from build123d import *

# Parameters (mm, degrees)
SKETCH1_W           = 127
SKETCH1_H           = 57.15
SKETCH1_R           = 14.3002
SKETCH1_R_2         = 2.38125
BOSS_EXTRUDE1_DEPTH = 3.175
SKETCH2_R           = 2.38125
CUT_EXTRUDE1_DEPTH  = 3.175
FILLET1_R           = 5.08
SKETCH3_R           = 3.175
CUT_EXTRUDE2_DEPTH  = 3.175
SKETCH4_R           = 16.51
CUT_EXTRUDE3_DEPTH  = 7.62
SKETCH5_W           = 76.2
SKETCH5_H           = 12.7
BOSS_EXTRUDE2_DEPTH = 3.175
FILLET2_R           = 5.08
SKETCH6_W           = 25.4
SKETCH6_H           = 5.08
BOSS_EXTRUDE3_DEPTH = 3.175
FILLET3_R           = 5.08
SKETCH7_R           = 2.38125
CUT_EXTRUDE4_DEPTH  = 3.175


with BuildPart() as part:
    # Sketch1 → Boss-Extrude1 (new body)
    with BuildSketch(Plane.XY):
        Rectangle(SKETCH1_W, SKETCH1_H)
        with Locations((31.75, 0)):
            Circle(SKETCH1_R, mode=Mode.SUBTRACT)
        with Locations((37.555148495, -24.727722316)):
            Circle(SKETCH1_R_2, mode=Mode.SUBTRACT)
        with Locations((10.16, 13.380280266)):
            Circle(SKETCH1_R_2, mode=Mode.SUBTRACT)
        with Locations((25.944851505, 24.727722316)):
            Circle(SKETCH1_R_2, mode=Mode.SUBTRACT)
        with Locations((53.34, -13.380280266)):
            Circle(SKETCH1_R_2, mode=Mode.SUBTRACT)
    extrude(amount=BOSS_EXTRUDE1_DEPTH)

    # Sketch2 → Cut-Extrude1 (cut)
    with BuildSketch(Plane.XY.offset(3.175)):
        with Locations((57.15, 22.225)):
            Circle(SKETCH2_R)
        with Locations((57.15, -22.225)):
            Circle(SKETCH2_R)
        with Locations((0, 22.225)):
            Circle(SKETCH2_R)
        with Locations((0, -22.225)):
            Circle(SKETCH2_R)
    extrude(amount=-CUT_EXTRUDE1_DEPTH, mode=Mode.SUBTRACT)

    # Fillet1
    fillet1_edges = [part.edges().sort_by_distance(p)[0] for p in [
        (63.5, -28.575, 1.5875),
        (63.5, 28.575, 1.5875),
    ]]
    fillet(fillet1_edges, radius=FILLET1_R)

    # Sketch3 → Cut-Extrude2 (cut)
    with BuildSketch(Plane.XY.offset(3.175)):
        with Locations((-57.15, 22.225)):
            Circle(SKETCH3_R)
        with Locations((-19.05, 22.225)):
            Circle(SKETCH3_R)
        with Locations(Location((-19.05, -22.225, 0), (0, 0, 180))):
            Circle(SKETCH3_R)
        with Locations(Location((-57.15, -22.225, 0), (0, 0, 180))):
            Circle(SKETCH3_R)
    extrude(amount=-CUT_EXTRUDE2_DEPTH, mode=Mode.SUBTRACT)

    # Sketch4 → Cut-Extrude3 (cut)
    with BuildSketch(Plane.XY.offset(3.175)):
        with Locations((-38.1, 9.525)):
            Circle(SKETCH4_R)
    extrude(amount=-CUT_EXTRUDE3_DEPTH, mode=Mode.SUBTRACT)

    # Sketch5 → Boss-Extrude2 (add)
    with BuildSketch(Plane.XY.offset(3.175)):
        with Locations((-50.8, -34.925)):
            Rectangle(SKETCH5_W, SKETCH5_H)
        with Locations((-50.8, 34.925)):
            Rectangle(SKETCH5_W, SKETCH5_H)
    extrude(amount=-BOSS_EXTRUDE2_DEPTH)

    # Fillet2
    fillet2_edges = [part.edges().sort_by_distance(p)[0] for p in [
        (-12.7, 41.275, 1.5875),
        (-12.7, 28.575, 1.5875),
        (-12.7, -28.575, 1.5875),
        (-12.7, -41.275, 1.5875),
    ]]
    fillet(fillet2_edges, radius=FILLET2_R)

    # Sketch6 → Boss-Extrude3 (add)
    with BuildSketch(Plane.XY.offset(3.175)):
        with Locations((-76.2, 26.035)):
            Rectangle(SKETCH6_W, SKETCH6_H)
    extrude(amount=-BOSS_EXTRUDE3_DEPTH)

    # Fillet3
    fillet3_edges = [part.edges().sort_by_distance(p)[0] for p in [
        (-88.9, 41.275, 1.5875),
        (-88.9, -41.275, 1.5875),
    ]]
    fillet(fillet3_edges, radius=FILLET3_R)

    # Sketch7 → Cut-Extrude4 (cut)
    with BuildSketch(Plane.XY.offset(3.175)):
        with Locations((-82.55, 34.925)):
            Circle(SKETCH7_R)
        with Locations((-82.55, -34.925)):
            Circle(SKETCH7_R)
        with Locations((-69.85, 34.925)):
            Circle(SKETCH7_R)
        with Locations((-69.85, -34.925)):
            Circle(SKETCH7_R)
    extrude(amount=-CUT_EXTRUDE4_DEPTH, mode=Mode.SUBTRACT)


solid = part.part
The listing builds one solid part. Answer for the finished solid, in the listing's coordinates (mm). Coordinates: 2 decimals unless noted, no trailing zeros. Loops run counter-clockwise (first coordinate to the right, second up) from the corner with the lowest first, then second, coordinate; pieces in that order, holes last.
1) Find section C-C on x = 31.75. Write down the section's boundary in (y, z) (3 decimals), then the cut area to 3 significant figures.
2) Flat-ended cylindrical pins translate along their axes: pin 1 Ø4 at (x, y) = (53.34, -13.38) entering from +Z; pin 2 Ø1.6 at (x, z) = (33.5, 1) entering from +Y (3 decimals). Find the tip coordinate at first contact, or state that the pin passes through.
3) Find the intervals of material crossed by L1, parallel to Y at x = -57.15, z = 2.4 (3 decimals); L2, parallel to Y at x = -69.85, z = 1.25 (3 decimals); L3, parallel to Y at x = 37, z = 2.85 (3 decimals), in increasing order.
4) Find section A-A on x = 10.16. Write down the section's boundary in (y, z) (3 decimals), then the cut area to 3 significant figures.
5) Determine the mould class of faces 1 (the face through (-84.93, -34.82, 1.61)), 2 (the face through (25, -28.575, 2)), 3 (the face through (-14.15, 39.75, 1.57)) for opening direction Y: pulls with the +Y half, pulls with the -Y half, needs draft (parallel to the pull), parting line crosses it, or undercut.
6) Find section B-B on y = -4. Write down the section's boundary in (x, z) (3 decimals), then the cut area to 3 significant figures.
7) Find section D-D on z = 1.9. Give the number of separate pieces and of enclosed holes in the cut face, then the cut area to 3 significant figures.
Values:
1. outline: (-28.575, 0) - (-14.3, 0) - (-14.3, 3.175) - (-28.575, 3.175) - close; (14.3, 0) - (28.575, 0) - (28.575, 3.175) - (14.3, 3.175) - close
1. area: 90.6 mm2
2. pin 1: passes through
2. pin 2: stops at y = 28.575
3. L1: y = -41.275 to -25.4, -19.05 to 19.05, 25.4 to 41.275
3. L2: y = -41.275 to -37.306, -32.544 to -28.575, 23.495 to 32.544, 37.306 to 41.275
3. L3: y = -28.575 to -27.043, -22.412 to -13.302, 13.302 to 28.575
4. outline: (-28.575, 0) - (10.999, 0) - (10.999, 3.175) - (-28.575, 3.175) - close; (15.762, 0) - (28.575, 0) - (28.575, 3.175) - (15.762, 3.175) - close
4. area: 166 mm2
5. face 1: undercut
5. face 2: pulls with the -Y half
5. face 3: pulls with the +Y half
6. outline: (-63.5, 0) - (-47.569, 0) - (-47.569, 3.175) - (-63.5, 3.175) - close; (-28.631, 0) - (18.021, 0) - (18.021, 3.175) - (-28.631, 3.175) - close; (45.479, 0) - (63.5, 0) - (63.5, 3.175) - (45.479, 3.175) - close
6. area: 256 mm2
7. separate pieces: 1
7. enclosed holes: 18
7. area: 7,460 mm2
